Design review of the part built by this model. Coordinates are the model's own, in mm. A direction names the side the tool comes from. Give positions to 0.01 mm unless a question says otherwise; leave off trailing zeros. Loops run counter-clockwise (first coordinate to the right, second up) from the corner with the lowest first, then second, coordinate; pieces in that order, holes last. Notation, with made-up numbers: M 61,-16.75 L 65,-16.75 A29 ccw 65,5.25 Z; hole C -40,83.25 d1. An arc over 180 degrees is marked long. Use a Markdown table: item, result. Add a question column.
(1) Add section A-A, the plane y = 115.5. Give the boundary of the cut face in (x, z).
(2) For faces 4 (the face through (87.275, 96.349, 12.325)), 5 (the face through (0, 25, 12)), list the 3-axis set-ups (+Z, -Z, +X, -X, +Y, -Y) from which the entire face can be reached by the end or side of a thin tool; tool diameter is ignored.
(3) Add section C-C, the plane x = -62.5. Give the boundary of the cut face in (y, z), then the cut area to 3 significant figures.
(4) Add section B-B, the plane x = -41. Give the boundary of the cut face in (y, z), then the cut area to 3 significant figures.
(5) For probe 1 along Y at (x, z) = (4, 10); probe 2 along Y at (x, z) = (13, 8.25); probe 3 along X at (y, z) = (83.5, 16.25), list the stretches that pass through material, from the lowest coordinate up.
(6) Add section D-D, the plane z = 9.75. Give the boundary of the cut face in (x, y).
(7) Draft analysis for pull direction Y (two halves, no side actions). For faces 1 (the face through (0, 8, 12)), 2 (the face through (-70.05, 89.51, 12.32)), 3 (the face through (-1, 70, 0)), state which applies: pulls with the +Y half, pulls with the -Y half, needs draft (parallel to the pull), parting line crosses it, or undercut.
(8) Insertion check: pin 1 Ø12 at (y, z) = (25.5, 10) entering from +X; pin 2 Ø5 at (x, z) = (-63.5, 18.5) entering from +Y; pin 3 Ø3 at (y, z) = (100, 19) entering from +X. Each pin has a flat end and moves straight along its axis. Give the tip position at first contact, or say it passes through.
```python
from build123d import *

# Parameters (mm, degrees)
F0_R     = 9
F1_DEPTH = 25


with BuildPart() as f1:
    # F0 (on Top) → F1 (new body)
    with BuildSketch(Plane.XY):
        with BuildLine():
            ThreePointArc((-24.100695, 156.899617), (-44.828984, 162.91459), (-57.806842, 145.668806))
            ThreePointArc((-57.806842, 145.668806), (-61.750067, 132.935178), (-71.485406, 123.829275))
            ThreePointArc((-71.485406, 123.829275), (-87.293644, 97.378424), (-71.450292, 70.948591))
            ThreePointArc((-71.450292, 70.948591), (-57.655484, 57.590544), (-52.98448, 38.964866))
            ThreePointArc((-52.98448, 38.964866), (-44.551636, 17.130716), (-23, 8))
            Line((-23, 8), (23, 8))
            ThreePointArc((23, 8), (44.551636, 17.130716), (52.98448, 38.964866))
            ThreePointArc((52.98448, 38.964866), (57.655484, 57.590544), (71.450292, 70.948591))
            ThreePointArc((71.450292, 70.948591), (87.287561, 96.793932), (72.504354, 123.256313))
            ThreePointArc((72.504354, 123.256313), (39.60509, 137.406102), (4.221762, 142.937667))
            ThreePointArc((4.221762, 142.937667), (-11.458365, 146.837486), (-24.100695, 156.899617))
        make_face()
        with BuildLine():
            Line((-23, 51), (22.999999, 51))
            ThreePointArc((22.999999, 51), (36, 38), (22.999999, 25))
            Line((22.999999, 25), (-23, 25))
            ThreePointArc((-23, 25), (-36, 38), (-23, 51))
        make_face(mode=Mode.SUBTRACT)
        with BuildLine():
            ThreePointArc((-49.688299, 84.469361), (-70.222634, 89.792993), (-64.899002, 110.327329))
            ThreePointArc((-64.899002, 110.327329), (0, 128), (64.899002, 110.327329))
            ThreePointArc((64.899002, 110.327329), (70.222634, 89.792993), (49.688299, 84.469361))
            ThreePointArc((49.688299, 84.469361), (0, 98), (-49.688299, 84.469361))
        make_face(mode=Mode.SUBTRACT)
        with Locations((-38.822857, 144.888874)):
            Circle(F0_R, mode=Mode.SUBTRACT)
    extrude(amount=F1_DEPTH)


solid = f1.part
```
Established:
| question | item | result |
|---|---|---|
| 1 | outline | M -81.22,0 L -55.17,0 L -55.17,25 L -81.22,25 Z; M 55.17,0 L 81.22,0 L 81.22,25 L 55.17,25 Z |
| 2 | face 4 | +Z, -Z, +X |
| 2 | face 5 | +Z, -Z |
| 3 | outline | M 64.1,0 L 83.33,0 L 83.33,25 L 64.1,25 Z; M 111.7,0 L 131.8,0 L 131.8,25 L 111.7,25 Z |
| 3 | area | 983 mm^2 |
| 4 | outline | M 14,0 L 89.01,0 L 89.01,25 L 14,25 Z; M 121.26,0 L 136.16,0 L 136.16,25 L 121.26,25 Z; M 153.62,0 L 163.76,0 L 163.76,25 L 153.62,25 Z |
| 4 | area | 2,500 mm^2 |
| 5 | probe 1 | 8 to 25, 51 to 97.92, 127.94 to 142.94 |
| 5 | probe 2 | 8 to 25, 51 to 97.13, 127.34 to 142.41 |
| 5 | probe 3 | -83.88 to -62.94, -51.65 to 51.65, 62.94 to 83.88 |
| 6 | outline | M -71.49,123.83 A30 ccw -71.45,70.95 A35 cw -52.98,38.96 A30 ccw -23,8 L 23,8 A30 ccw 52.98,38.96 A35 cw 71.45,70.95 A30 ccw 72.5,123.26 A143 ccw 4.22,142.94 A38 cw -24.1,156.9 A19 ccw -57.81,145.67 A26 cw Z; hole M -64.9,110.33 A15 ccw -49.69,84.47 A98 cw 49.69,84.47 A15 ccw 64.9,110.33 A128 ccw Z; hole C -38.82,144.89 d18; hole M -23,25 L 23,25 A13 ccw 23,51 L -23,51 A13 ccw Z |
| 7 | face 1 | pulls with the -Y half |
| 7 | face 2 | undercut |
| 7 | face 3 | needs draft |
| 8 | pin 1 | x = 52.29 |
| 8 | pin 2 | y = 134.21 |
| 8 | pin 3 | x = 87.27 |
